```python
from build123d import *

# Parameters (mm, degrees)
F1_DEPTH = 19.05
F3_DEPTH = 8.4666582
F5_DEPTH = 9.525


# Not quite as in the source:
# - a feature names something its author has since deleted; it is built from what else it names


with BuildPart() as f1:
    # F0 (on Top) → F1 (new body)
    with BuildSketch(Plane.XY):
        with BuildLine():
            Line((727.2677384075, 427.9083177516), (727.2677384075, -283.5772421425))
            ThreePointArc((727.2677384075, -283.5772421425), (774.4074471785, -328.2362889839), (816.4554812019, -278.7535097314))
            Line((816.4554812019, -278.7535097314), (816.4554812019, -221.0955097314))
            Line((816.4554812019, -221.0955097314), (1159.4623036636, -98.9686407408))
            Line((1159.4623036636, -98.9686407408), (1178.6487772739, -128.0367093729))
            Line((1178.6487772739, -128.0367093729), (1189.3036458742, -145.3996676047))
            ThreePointArc((1189.3036458742, -145.3996676047), (1254.3589120262, -165.180351508), (1280.8355912672, -102.5508970465))
            Line((1280.8355912672, -102.5508970465), (881.2480453078, 396.8848219998))
            ThreePointArc((881.2480453078, 396.8848219998), (878.9075846932, 401.4943033077), (878.5980767553, 406.6546597539))
            Line((878.5980767553, 406.6546597539), (902.2401524871, 568.497452094))
            ThreePointArc((902.2401524871, 568.497452094), (903.8120375637, 573.0182606597), (906.9455405898, 576.6362285378))
            Line((906.9455405898, 576.6362285378), (941.9003890149, 604.1852707886))
            Line((941.9003890149, 604.1852707886), (899.3018677789, 723.8279303566))
            Line((899.3018677789, 723.8279303566), (891.7270738587, 721.1309406639))
            Line((891.7270738587, 721.1309406639), (888.532184766, 730.1041401315))
            Line((888.532184766, 730.1041401315), (557.8398737201, 612.361827435))
            Line((557.8398737201, 612.361827435), (561.0347628128, 603.3886279674))
            Line((561.0347628128, 603.3886279674), (540.3738890749, 596.0323666485))
            Line((540.3738890749, 596.0323666485), (579.8650741531, 488.7713005475))
            ThreePointArc((579.8650741531, 488.7713005475), (586.4584656719, 481.6292642269), (596.1708798397, 481.2413137672))
            Line((596.1708798397, 481.2413137672), (710.1798289544, 523.2169221936))
            ThreePointArc((710.1798289544, 523.2169221936), (721.8328450807, 521.7157540947), (727.2677384075, 511.2990259602))
            Line((727.2677384075, 511.2990259602), (727.2677384075, 427.9083177516))
        make_face()
        with BuildLine():
            Line((1099.3852571882, -15.0422832395), (825.3589785984, -112.6087723988))
            Line((825.3589785984, -112.6087723988), (812.2279623998, 291.9047427935))
            ThreePointArc((812.2279623998, 291.9047427935), (820.3847868922, 304.1789193457), (834.6503380579, 300.4798321914))
            Line((834.6503380579, 300.4798321914), (1099.3852571882, -15.0422832395))
        make_face(mode=Mode.SUBTRACT)
    extrude(amount=F1_DEPTH)

    # F2 (on face) → F3 (cut)
    with BuildSketch(Plane.XY.offset(19.05)):
        with BuildLine():
            ThreePointArc((838.451528287, -152.2525984903), (831.9027765287, -166.0430988586), (845.6932768971, -172.5918506169))
            Line((845.6932768971, -172.5918506169), (1132.8356598603, -70.3553996504))
            ThreePointArc((1132.8356598603, -70.3553996504), (1139.3844116185, -56.564899282), (1125.5939112501, -50.0161475238))
            Line((1125.5939112501, -50.0161475238), (838.451528287, -152.2525984903))
        make_face()
    extrude(amount=-F3_DEPTH, mode=Mode.SUBTRACT)

    # F4 (on face) → F5 (cut)
    with BuildSketch(Plane.XY.offset(19.05)):
        Polygon((579.7007303012, 517.0436017545), (586.2609025716, 498.618632181), (926.4367371726, 619.7375338049), (930.6009060633, 621.2201775171), (924.161381266, 639.3062953154), (919.9972123753, 637.8236516032), (891.8491444715, 716.8806143331), (890.4923506062, 720.6913200061), (891.7270738587, 721.1309406639), (888.532184766, 730.1041401315), (869.645537074, 723.3795883228), (874.197220032, 710.5956831823), (902.2246404628, 631.8775722275), align=None)
    extrude(amount=-F5_DEPTH, mode=Mode.SUBTRACT)


solid = f1.part
```
Part model, mm, in its own coordinate system. A direction names the side the tool comes from. Give positions to 0.01 mm unless a question says otherwise; leave off trailing zeros. Loops run counter-clockwise (first coordinate to the right, second up) from the corner with the lowest first, then second, coordinate; pieces in that order, holes last. Notation, with made-up numbers: M 41.5,73.5 L 49.5,73.5 A15 ccw 49.5,90.5 Z; hole C 78.25,-40 d7. An arc over 180 degrees is marked long. Return JSON: item names as keys, results as strings.
1) 3-axis set-ups, long thin cutter, end or side, ignore diameter. For faces 1 (the face through (793, 589, 9.525)), 2 (the face through (964.29, -63.143, 9.392)), 3 (the face through (890.254, 486.443, 9.392)): which of +Z, -Z, +X, -X, +Y, -Y reach the whole face in a straight line?
Calculated:
{"face 1": "+Z", "face 2": "+Z, -Z", "face 3": "+Z, -Z, +X"}
2) Saw through at B-B, the plane z = 4.25. List the corners of the cut face in (x, y), then the cut area to 3 significant figures.
Calculated:
{"outline": "M 540.37,596.03 L 579.87,488.77 A12.7 ccw 596.17,481.24 L 710.18,523.22 A12.7 cw 727.27,511.3 L 727.27,-283.58 A44.72 ccw long 816.46,-278.75 L 816.46,-221.1 L 1159.46,-98.97 L 1178.65,-128.04 L 1189.3,-145.4 A50.81 ccw 1280.84,-102.55 L 881.25,396.88 A12.7 cw 878.6,406.65 L 902.24,568.5 A12.7 cw 906.95,576.64 L 941.9,604.19 L 899.3,723.83 L 891.73,721.13 L 888.53,730.1 L 557.84,612.36 L 561.03,603.39 Z; hole M 812.23,291.9 L 825.36,-112.61 L 1099.39,-15.04 L 834.65,300.48 A12.7 ccw Z", "area": "239,000 mm2"}
3) Saw through at A-A, the plane y = 91. List the corners of the cut face in (x, z).
Calculated:
{"outline": "M 727.27,0 L 818.75,0 L 818.75,19.05 L 727.27,19.05 Z; M 1010.41,0 L 1125.98,0 L 1125.98,19.05 L 1010.41,19.05 Z"}
4) Pull direction Y, two halves, no side cores. Call faces 4 (the face through (725.501, 672.057, 9.392)), 5 (the face through (965.16, 144.93, 9.39)), 6 (the face through (652.377, 501.935, 9.392)): released by +Y, released by -Y, zero draft, split by the parting line, or undercut.
Calculated:
{"face 4": "released by +Y", "face 5": "undercut", "face 6": "released by -Y"}
5) Saw through at D-D, the plane x = 630. List the corners of the cut face in (y, z) (3 decimals).
Calculated:
{"outline": "M 493.696,0 L 638.054,0 L 638.054,19.05 L 534.953,19.05 L 534.953,9.525 L 514.192,9.525 L 514.192,19.05 L 493.696,19.05 Z"}
6) Flat gauge pins, fed straight in: pin 1 Ø8 at (y, z) = (234, 17) entering from +X; pin 2 Ø2 at (x, z) = (1110.5, 8.5) entering from -Y; pin 3 Ø3 at (x, z) = (722.5, 7) entering from +Y. Where does each tip first touch, or does it go through?
Calculated:
{"pin 1": "stops at x = 1014.77", "pin 2": "stops at y = -116.76", "pin 3": "stops at y = 671.52"}
7) Drill centre lines: line 1 (Y direction, x = 947.5, z = 12.5); line 2 (Y direction, x = 979.5, z = 18); line 3 (X direction, y = -250, z = 7.5). Where is each one in solid material? Low to high.
Calculated:
{"line 1": "y = -174.44 to -136.34, -113.43 to -69.12, 165.98 to 314.08", "line 2": "y = -163.04 to -124.95, -102.03 to -57.73, 127.84 to 274.08", "line 3": "x = 727.27 to 816.46"}
8) Saw through at C-C, the plane x = 1059.5. List the corners of the cut face in (y, z).
Calculated:
{"outline": "M -134.56,0 L -29.24,0 L -29.24,19.05 L -73.55,19.05 L -73.55,10.58 L -96.47,10.58 L -96.47,19.05 L -134.56,19.05 Z; M 32.49,0 L 174.09,0 L 174.09,19.05 L 32.49,19.05 Z"}
